from build123d import *

# Parameters (mm, degrees)
F0_DEPTH = 12.7
F1_W     = 5.08
F1_H     = 2.54
F2_DEPTH = 2.54


with BuildPart() as f0:
    # F3 (on Front) → F0 (new body)
    with BuildSketch(Plane.XZ):
        with BuildLine():
            Line((-31.361033, 69.238202), (-50.411033, 69.238202))
            Line((-50.411033, 69.238202), (-50.411033, 35.634632))
            ThreePointArc((-50.411033, 35.634632), (-40.886033, 37.488202), (-31.361033, 35.634632))
            Line((-31.361033, 35.634632), (-31.361033, 69.238202))
        make_face()
        with BuildLine():
            ThreePointArc((-31.361033, 35.634632), (-40.886033, 37.488202), (-50.411033, 35.634632))
            Line((-50.411033, 35.634632), (-50.411033, 12.088202))
            Line((-50.411033, 12.088202), (-31.361033, 12.088202))
            Line((-31.361033, 12.088202), (-31.361033, 35.634632))
        make_face()
        with BuildLine():
            Line((-50.411033, 12.088202), (-50.411033, 35.634632))
            ThreePointArc((-50.411033, 35.634632), (-55.085064, -8.972365), (-15.486033, 12.088202))
            ThreePointArc((-15.486033, 12.088202), (-19.825465, 26.287234), (-31.361033, 35.634632))
            Line((-31.361033, 35.634632), (-31.361033, 12.088202))
            Line((-31.361033, 12.088202), (-50.411033, 12.088202))
        make_face()
    extrude(amount=F0_DEPTH)

    # F1 (on face) → F2 (join)
    with BuildSketch(Plane.XY.offset(69.238202)):
        with Locations((-40.886033, -6.35)):
            Rectangle(F1_W, F1_H)
    extrude(amount=F2_DEPTH)


solid = f0.part
The listing builds one solid part. Answer for the finished solid, in the listing's coordinates (mm). A direction names the side the tool comes from. Give positions to 0.01 mm unless a question says otherwise; leave off trailing zeros. Write each loop counter-clockwise with the first axis right and the second up, starting at its lowest first coordinate (ties: lowest second). Pieces come first, ordered by that corner, then holes.
1) Section B-B (x = -25) is taken. Write down the section's boundary in (y, z).
2) Find the intervals of material crossed by L1, parallel to Z at x = -41, y = -10.25; L2, parallel to Z at x = -29, y = -5; L3, parallel to X at y = -0.5, z = 11.5, in increasing order.
3) Section D-D (y = -3) is taken. Write down the section's boundary in (x, z).
4) Section A-A (y = -6.75) is taken. Write down the section's boundary in (x, z).
5) A tool of negligible diameter and unlimited length cuts with its end or side. For faces 1 (the face through (-38.346, -6, 70)), 2 (the face through (-50.411, -6, 53)), 3 (the face through (-41, -6, 71.778)), 4 (the face through (-41, -5.08, 70)), 5 (the face through (-41, -7.62, 70)), from which of +Z, -Z, +X, -X, +Y, -Y can it reach the whole face along a straight path? Write none if from no direction.
6) Given P1, Ø4, axis at y = -8, z = 46, coming from the +X side; P2, Ø6, axis at y = -6.5, z = 58, coming from the -X side; P3, Ø0.8, axis at y = -6.5, z = 70.5, coming from the -X side, each flat-ended and moving along its own axis, determine where each tip first touches the part or whether it passes through.
7) Section C-C (z = 50) is taken. Write down the section's boundary in (x, y), and give its area (3 significant figures).
Response:
1. outline: (-12.7, -7.73) - (0, -7.73) - (0, 31.91) - (-12.7, 31.91) - close
2. L1: z = -13.31 to 69.24
2. L2: z = -10.36 to 34.54
2. L3: x = -66.28 to -15.49
3. outline: (-50.41, 35.63) arc R25.4 ccw (long way) to (-15.49, 12.09) arc R25.4 ccw to (-31.36, 35.63) - (-31.36, 69.24) - (-50.41, 69.24) - close
4. outline: (-50.41, 35.63) arc R25.4 ccw (long way) to (-15.49, 12.09) arc R25.4 ccw to (-31.36, 35.63) - (-31.36, 69.24) - (-38.35, 69.24) - (-38.35, 71.78) - (-43.43, 71.78) - (-43.43, 69.24) - (-50.41, 69.24) - close
5. face 1: +Z, +X, +Y, -Y
5. face 2: +Z, -X, +Y, -Y
5. face 3: +Z, +X, -X, +Y, -Y
5. face 4: +Z, +X, -X, +Y
5. face 5: +Z, +X, -X, -Y
6. P1: stops at x = -31.36
6. P2: stops at x = -50.41
6. P3: stops at x = -43.43
7. outline: (-50.41, -12.7) - (-31.36, -12.7) - (-31.36, 0) - (-50.41, 0) - close
7. area: 242 mm2
